from build123d import *

# Parameters (mm, degrees)
F0_W     = 114.3
F0_H     = 114.3
F0_R     = 50.8
F1_DEPTH = 3.175
F2_W     = 114.3
F2_H     = 3.175
F3_DEPTH = 12.7
F5_DEPTH = 25.4


with BuildPart() as f1:
    # F0 (on Front) → F1 (new body)
    with BuildSketch(Plane.XZ):
        Rectangle(F0_W, F0_H)
        Circle(F0_R, mode=Mode.SUBTRACT)
    extrude(amount=F1_DEPTH)

    # F2 (on face) → F3 (join)
    with BuildSketch(Plane.XZ.offset(3.175)):
        with Locations((0, 55.5625)):
            Rectangle(F2_W, F2_H)
    extrude(amount=F3_DEPTH)

    # F4 (on face) → F5 (cut)
    with BuildSketch(Plane.XY.offset(57.15)):
        with BuildLine():
            ThreePointArc((-41.275, -7.9375), (-44.45, -4.7625), (-47.625, -7.9375))
            Line((-47.625, -7.9375), (-41.275, -7.9375))
        make_face()
        with BuildLine():
            ThreePointArc((47.625, -7.9375), (44.45, -4.7625), (41.275, -7.9375))
            Line((41.275, -7.9375), (47.625, -7.9375))
        make_face()
        with BuildLine():
            Line((47.625, -7.9375), (41.275, -7.9375))
            ThreePointArc((41.275, -7.9375), (44.45, -11.1125), (47.625, -7.9375))
        make_face()
        with BuildLine():
            ThreePointArc((3.175, -7.9375), (0, -4.7625), (-3.175, -7.9375))
            Line((-3.175, -7.9375), (3.175, -7.9375))
        make_face()
        with BuildLine():
            Line((3.175, -7.9375), (-3.175, -7.9375))
            ThreePointArc((-3.175, -7.9375), (0, -11.1125), (3.175, -7.9375))
        make_face()
        with BuildLine():
            Line((-41.275, -7.9375), (-47.625, -7.9375))
            ThreePointArc((-47.625, -7.9375), (-44.45, -11.1125), (-41.275, -7.9375))
        make_face()
    extrude(amount=-F5_DEPTH, mode=Mode.SUBTRACT)


solid = f1.part
Here's how the part is built. I have some questions about the finished solid (model axes, mm). A direction names the side the tool comes from. Give positions to 0.01 mm unless a question says otherwise; leave off trailing zeros. Order: outer loops, then holes, each group sorted by start corner. A loop starts at its lowest first (then second) coordinate and runs counter-clockwise, first axis right, second up. Notation, with made-up numbers: M 87,-29 L 128,-29 A19 ccw 128,-23 Z; hole C 18.5,56.5 d4. An arc over 180 degrees is marked long. Answer as a JSON object with one key per item and string values. Group by question number.
1) On a 3-axis mill with a long thin cutter (end or side, diameter ignored), from which of +Z, -Z, +X, -X, +Y, -Y can I reach the whole of each face in a straight line? I mean faces 1 (the cylindrical face through (0.413, -11.085, 55.585)), 2 (the flat face through (-1, -12, 53.975)). Say none if no direction works.
2) Please list where these lines run through material, in increasing order: L1, parallel to Y at x = 0, z = 55 (1 decimal); L2, parallel to Z at x = 0, y = -1.6; L3, parallel to Z at x = -10, y = -8.25 (3 decimals). Write a range as [from, to].
3) Suppose I cut it at C-C, the plane y = -9.25. Write out the boundary of the cut face in (x, z) (3 decimals), plus the area to 3 significant figures.
4) Suppose I cut it at A-A, the plane z = 0. Write out the boundary of the cut face in (x, y) (3 decimals), plus the area to 3 significant figures.
5) I'm going to push a flat-ended pin straight in: pin 1 Ø5.5 at (x, y) = (-44.45, -7.94) entering from +Z. Where does the tip first touch, or does it pass through?
6) We'd pull the mould along Y, two halves only. Please class faces 3 (the flat face through (-52, 0, 1)), 4 (the cylindrical face through (-41.28, -8.08, 55.58)), 5 (the flat face through (57.15, -3, 8)), 6 (the flat face through (-14, -3.175, -50)): pulls with the +Y half, pulls with the -Y half, needs draft (parallel to the pull), parting line crosses it, or undercut.
7) Suppose I cut it at B-B, the plane x = 44.45. Count the separate pieces of the cut face and the enclosed holes in it, plus the area to 3 significant figures.
8) Suppose I cut it at D-D, the plane x = -35. Write out the boundary of the cut face in (y, z) (3 decimals).
Results found:
{
 "1": {"face 1": "+Z, -Z", "face 2": "-Z, +X, -X, -Y"},
 "2": {"L1": "[-15.9, -11.1], [-4.8, 0]", "L2": "[-57.15, -50.8], [50.8, 57.15]", "L3": "[53.975, 57.15]"},
 "3": {"outline": "M -57.15,53.975 L -47.341,53.975 L -47.341,57.15 L -57.15,57.15 Z; M -41.559,53.975 L -2.891,53.975 L -2.891,57.15 L -41.559,57.15 Z; M 2.891,53.975 L 41.559,53.975 L 41.559,57.15 L 2.891,57.15 Z; M 47.341,53.975 L 57.15,53.975 L 57.15,57.15 L 47.341,57.15 Z", "area": "308 mm²"},
 "4": {"outline": "M -57.15,-3.175 L -50.8,-3.175 L -50.8,0 L -57.15,0 Z; M 50.8,-3.175 L 57.15,-3.175 L 57.15,0 L 50.8,0 Z", "area": "40.3 mm²"},
 "5": {"pin 1": "through"},
 "6": {"face 3": "pulls with the +Y half", "face 4": "undercut", "face 5": "needs draft", "face 6": "pulls with the -Y half"},
 "7": {"separate pieces": "3", "enclosed holes": "0", "area": "227 mm²"},
 "8": {"outline": "M -15.875,53.975 L -3.175,53.975 L -3.175,36.819 L 0,36.819 L 0,57.15 L -15.875,57.15 Z; M -3.175,-57.15 L 0,-57.15 L 0,-36.819 L -3.175,-36.819 Z"}
}
